Work out the finished part from the listing and answer in its coordinate system (mm). A direction names the side the tool comes from. Coordinates: 2 decimals unless noted, no trailing zeros. Write each loop counter-clockwise with the first axis right and the second up, starting at its lowest first coordinate (ties: lowest second). Pieces come first, ordered by that corner, then holes. Notation, with made-up numbers: (87, -38) - (137, -38) arc R17 cw to (137, -9) - close; hole circle Ø4 at (82, 74.5). An arc over 180 degrees is marked (long way). Use one line per item in the form item = value. Start each with the question number.
Item 1: For faces 1 (the cylindrical face through (-7.75, 0.01, 1.48)), 2 (the cylindrical face through (-5.49, -5.47, 1.48)), determine the directions among +Z, -Z, +X, -X, +Y, -Y from which every point of the face is accessible in a straight line to the end or side of a thin tool.
Item 2: Given pin 1 (1 mm diameter, centred on y = -3, z = 1, fed in from -X); pin 2 (1.5 mm diameter, centred on y = 7.5, z = 2, fed in from +X), each flat-ended and moving along its own axis, determine where each tip first touches the part or whether it passes through.
Item 3: Determine the mould class of faces 3 (the flat face through (-2, 2, 0)), 4 (the cylindrical face through (5.49, 5.47, 1.48)), 5 (the cylindrical face through (-0.01, -7.75, 1.48)) for opening direction Y: released by +Y, released by -Y, zero draft, split by the parting line, or undercut.
Item 4: Consider probe 1 along Y at (x, z) = (0, 1.8); probe 2 along X at (y, z) = (8, 2.05); probe 3 along X at (y, z) = (-7, 2.5). Determine where each line is inside the solid, lowest interval first.
Item 5: A cutting plane is placed at A-A (x = 0). Write down the section's boundary in (y, z).
Item 6: A cutting plane is placed at C-C (y = 2.75). Write down the section's boundary in (x, z).
from build123d import *

# Parameters (mm, degrees)
SKETCH1_R           = 9.5
SKETCH1_R_2         = 2.45
BOSS_EXTRUDE1_DEPTH = 3
CUT_EXTRUDE1_DEPTH  = 10
CIRPATTERN1_COUNT   = 16


with BuildPart() as part:
    # Sketch1 → Boss-Extrude1 (new body)
    with BuildSketch(Plane.XY):
        Circle(SKETCH1_R)
        Circle(SKETCH1_R_2, mode=Mode.SUBTRACT)
    extrude(amount=BOSS_EXTRUDE1_DEPTH)

    # Sketch6 → Cut-Extrude1 (cut)
    with BuildSketch(Plane(origin=(0, 0, 0), x_dir=(-1, 0, 0), z_dir=(0, 0, -1))):
        with BuildLine():
            ThreePointArc((-0.6, 7.726739286), (0, 7.75), (0.6, 7.726739286))
            add(Edge.make_bspline(
                [(1.495318178, 9.381578947), (1.036824569, 8.853460115), (0.705300974, 8.349634332), (0.6, 7.726739286)],
                knots=[0, 0, 0, 0, 1, 1, 1, 1], degree=3))
            ThreePointArc((1.495318178, 9.381578947), (0, 9.5), (-1.495318178, 9.381578947))
            add(Edge.make_bspline(
                [(-1.495318178, 9.381578947), (-1.036824569, 8.853460115), (-0.705300974, 8.349634332), (-0.6, 7.726739286)],
                knots=[0, 0, 0, 0, 1, 1, 1, 1], degree=3))
        make_face()
    cut_extrude1 = extrude(amount=-CUT_EXTRUDE1_DEPTH, mode=Mode.SUBTRACT)

    # CirPattern1: Cut-Extrude1 ×16 about axis
    cirpattern1_axis = Axis((0, 0, 0), (0, 0, 1))
    for i in range(1, CIRPATTERN1_COUNT):
        add(cut_extrude1.rotate(cirpattern1_axis, i * 360 / CIRPATTERN1_COUNT), mode=Mode.SUBTRACT)


solid = part.part
Answer:
q1.face_1 = +Z, -Z, -X
q1.face_2 = +Z, -Z
q2.pin_1 = -7.34
q2.pin_2 = 5.58
q3.face_3 = zero draft
q3.face_4 = undercut
q3.face_5 = released by -Y
q4.probe_1 = -7.75 to -2.45, 2.45 to 7.75
q4.probe_2 = -5.12 to -4.79, -2.46 to -0.66, 0.66 to 2.46, 4.79 to 5.12
q4.probe_3 = -5.49 to -3.57, -3.33 to 3.33, 3.57 to 5.49
q5.outline = (-7.75, 0) - (-2.45, 0) - (-2.45, 3) - (-7.75, 3) - close; (2.45, 0) - (7.75, 0) - (7.75, 3) - (2.45, 3) - close
q6.outline = (-7.25, 0) - (7.25, 0) - (7.25, 3) - (-7.25, 3) - close
